from build123d import *

# Parameters (mm, degrees)
SKETCH_1_W          = 20
SKETCH_1_H          = 70
SKETCH_1_R          = 1.5
SKETCH_1_W_2        = 6
SKETCH_1_H_2        = 52
EXTRUDE_1_DEPTH     = 2
SKETCH_2_W          = 0.5
SKETCH_2_H          = 26
CUT_EXTRUDE_1_DEPTH = 37.455452267
EXTRUDE_3_DEPTH     = 2
SKETCH_4_W          = 11.4
SKETCH_4_H          = 27.4
SKETCH_4_W_2        = 9
SKETCH_4_H_2        = 25
EXTRUDE_4_DEPTH     = 15
DRAFT_START         = -16.7
DRAFT_1_DEPTH       = 11.4
DRAFT_START_2       = -13.235626686
DRAFT_1_2_DEPTH     = 13.235626686


with BuildPart() as part:
    # Эскиз1 → Бобышка-Вытянуть1 (new body)
    with BuildSketch(Plane(origin=(0, 0, 0), x_dir=(1, 0, 0), z_dir=(0, 1, 0))):
        Rectangle(SKETCH_1_W, SKETCH_1_H)
        with Locations(Location((0, 30, 0), (0, 0, 270))):
            Circle(SKETCH_1_R, mode=Mode.SUBTRACT)
        with Locations(Location((0, -30, 0), (0, 0, 270))):
            Circle(SKETCH_1_R, mode=Mode.SUBTRACT)
        Rectangle(SKETCH_1_W_2, SKETCH_1_H_2, mode=Mode.SUBTRACT)
    extrude(amount=EXTRUDE_1_DEPTH)

    # Эскиз2 → Вырез-Вытянуть1 (cut, through all)
    with BuildSketch(Plane(origin=(0, 2, 0), x_dir=(1, 0, 0), z_dir=(0, 1, 0))):
        with Locations((-3.25, -13)):
            Rectangle(SKETCH_2_W, SKETCH_2_H)
        with Locations((-3.25, 13)):
            Rectangle(SKETCH_2_W, SKETCH_2_H)
        with BuildLine():
            ThreePointArc((4, 30), (2.828427125, 27.171572875), (0, 26))
            Line((0, 26), (3, 26))
            Line((3, 26), (3, 0))
            Line((3, 0), (10, 0))
            Line((10, 0), (10, 35))
            Line((10, 35), (-1.801814511, 35))
            ThreePointArc((-1.801814511, 35), (-2.371833534, 34.50465844), (-2.933620688, 34))
            Line((-2.933620688, 34), (0, 34))
            ThreePointArc((0, 34), (2.828427125, 32.828427125), (4, 30))
        make_face()
        with BuildLine():
            ThreePointArc((-10, 27.658633372), (-7.367393186, 30.953957731), (-4.449961479, 34))
            ThreePointArc((-4.449961479, 34), (-3.913284985, 34.504235123), (-3.368774283, 35))
            Line((-3.368774283, 35), (-10, 35))
            Line((-10, 35), (-10, 27.658633372))
        make_face()
        with BuildLine():
            Line((10, 0), (3, 0))
            Line((3, 0), (3, -26))
            Line((3, -26), (0, -26))
            ThreePointArc((0, -26), (2.828427125, -27.171572875), (4, -30))
            ThreePointArc((4, -30), (1.336481718, -33.770121565), (-3.106908308, -32.519349274))
            Line((-3.106908308, -32.519349274), (-4.5, -30.80136273))
            Line((-4.5, -30.80136273), (-4.5, -32.5))
            ThreePointArc((-4.5, -32.5), (-3.175976694, -33.777056798), (-1.801814511, -35))
            Line((-1.801814511, -35), (10, -35))
            Line((10, -35), (10, 0))
        make_face()
        with BuildLine():
            Line((-4.5, -32.5), (-4.5, -30.80136273))
            Line((-4.5, -30.80136273), (-10, -24.018660595))
            Line((-10, -24.018660595), (-10, -35))
            Line((-10, -35), (-1.801814511, -35))
            ThreePointArc((-1.801814511, -35), (-3.175976694, -33.777056798), (-4.5, -32.5))
        make_face()
    extrude(amount=-CUT_EXTRUDE_1_DEPTH, mode=Mode.SUBTRACT)

    # Эскиз3 → Бобышка-Вытянуть3 (add)
    with BuildSketch(Plane(origin=(0, 2, 0), x_dir=(1, 0, 0), z_dir=(0, 1, 0))):
        with BuildLine():
            Line((-15.931618932, -16.703677979), (-10, -24.018660595))
            Line((-10, -24.018660595), (-10, 27.658633372))
            ThreePointArc((-10, 27.658633372), (-18.585418451, 6.228867289), (-15.931618932, -16.703677979))
        make_face()
    extrude(amount=-EXTRUDE_3_DEPTH)

    # Эскиз4 → Бобышка-Вытянуть4 (add)
    with BuildSketch(Plane.XZ):
        with Locations((-11, 0)):
            Rectangle(SKETCH_4_W, SKETCH_4_H)
        with Locations((-11, 0)):
            Rectangle(SKETCH_4_W_2, SKETCH_4_H_2, mode=Mode.SUBTRACT)
    extrude(amount=EXTRUDE_4_DEPTH)

    # Уклон1: read off the stored shape, not the designer's step
    # Уклон1 outline → Уклон1 (add)
    with BuildSketch(Plane.YZ.offset(DRAFT_START)):
        Polygon((0, 13.7), (0, 20.694614872), (-15, 13.7), align=None)
        Polygon((0, -20.694614872), (0, -13.7), (-15, -13.7), align=None)
    extrude(amount=DRAFT_1_DEPTH)

    # Draft 1 2 outline → Draft 1 2 (cut)
    with BuildSketch(Plane(origin=(0, 0, 0), x_dir=(1, 0, 0), z_dir=(0, 1, 0)).offset(DRAFT_START_2)):
        with BuildLine():
            Line((-11.63690415, -22), (-15.931618932, -16.703677979))
            ThreePointArc((-15.931618932, -16.703677979), (-16.329223887, -15.617935511), (-16.7, -14.522740789))
            Line((-16.7, -14.522740789), (-16.7, -22))
            Line((-16.7, -22), (-11.63690415, -22))
        make_face()
        with BuildLine():
            Line((-16.7, 22), (-16.7, 14.522740788))
            ThreePointArc((-16.7, 14.522740788), (-15.2783441, 18.329891761), (-13.533119315, 22))
            Line((-13.533119315, 22), (-16.7, 22))
        make_face()
    extrude(amount=DRAFT_1_2_DEPTH, mode=Mode.SUBTRACT)


solid = part.part
The listing builds one solid part. Answer for the finished solid, in the listing's coordinates (mm). A direction names the side the tool comes from. Coordinates: 2 decimals unless noted, no trailing zeros. Loops run counter-clockwise (first coordinate to the right, second up) from the corner with the lowest first, then second, coordinate; pieces in that order, holes last.
1) A tool of negligible diameter and unlimited length cuts with its end or side. For faces 4 (the face through (-15.5, -7, 0)), 5 (the face through (-18, 0, 0)), 6 (the face through (-5.3, -8, 0)), from which of +Z, -Z, +X, -X, +Y, -Y can it reach the whole face along a straight path? Write none if from no direction.
2) Find section A-A on y = -11. Write down the section's boundary in (x, z), then the cut area to 3 significant figures.
3) Find section B-B on x = -7.25. Write down the section's boundary in (y, z), then the cut area to 3 significant figures.
4) Find section C-C on z = -7. Write down the section's boundary in (x, y).
5) Find the intervals of material crossed by L1, parallel to X at y = -4, z = -2; L2, parallel to Y at x = -5.25, z = -25; L3, parallel to X at y = 0.5, z = -14.5, in increasing order.
6) Determine the mould class of faces 1 (the face through (-3, 1, -35)), 2 (the face through (-11, -7, -12.5)), 3 (the face through (-4, 0, -6)) for opening direction Z: pulls with the +Z half, pulls with the -Z half, needs draft (parallel to the pull), parting line crosses it, or undercut.
7) Find section D-D on y = -1. Write down the section's boundary in (x, z).
8) Flat-ended cylindrical pins translate along their axes: pin 1 Ø5 at (x, y) = (-5.5, -5) entering from -Z; pin 2 Ø4.5 at (x, y) = (-9.5, -7) entering from +Z; pin 3 Ø1 at (y, z) = (0.5, 3.5) entering from +X. Find the tip coordinate at first contact, or state that the pin passes through.
Values:
1. face 4: -Y
1. face 5: +Z, -Z, -X, -Y
1. face 6: +Z, -Z, +X, -Y
2. outline: (-16.7, -14.52) arc R47 ccw to (-16.35, -15.57) - (-5.3, -15.57) - (-5.3, 15.57) - (-16.35, 15.57) arc R47 ccw to (-16.7, 14.52) - close; hole (-15.5, -12.5) - (-6.5, -12.5) - (-6.5, 12.5) - (-15.5, 12.5) - close
2. area: 130 mm2
3. outline: (-15, -13.7) - (0, -20.69) - (0, -31.09) - (2, -31.09) - (2, 27.41) - (0, 27.41) - (0, 20.69) - (-15, 13.7) - (-15, 12.5) - (0, 12.5) - (0, -12.5) - (-15, -12.5) - close
3. area: 258 mm2
4. outline: (-18.48, 0) - (-16.7, 0) - (-16.7, -15) - (-15.5, -15) - (-15.5, 0) - (-6.5, 0) - (-6.5, -15) - (-5.3, -15) - (-5.3, 0) - (-3.5, 0) - (-3.5, 2) - (-18.48, 2) - close
5. L1: x = -16.7 to -15.5, -6.5 to -5.3
5. L2: y = 0 to 2
5. L3: x = -16.71 to -3.5
6. face 1: pulls with the -Z half
6. face 2: undercut
6. face 3: needs draft
7. outline: (-16.7, -14.52) arc R47 ccw to (-14.42, -20.23) - (-5.3, -20.23) - (-5.3, 20.23) - (-13.07, 20.23) - (-15.93, 16.7) arc R47 ccw to (-16.7, 14.52) - close; hole (-15.5, -12.5) - (-6.5, -12.5) - (-6.5, 12.5) - (-15.5, 12.5) - close
8. pin 1: stops at z = -19.53
8. pin 2: stops at z = 18.48
8. pin 3: stops at x = -3.5
